Can you work these out from the model? Positions are in its coordinate system, mm. Face numbers are marked on the shaded views. A direction names the side the tool comes from. Round coordinates to 2 decimals unless told otherwise and drop trailing zeros. Order: outer loops, then holes, each group sorted by start corner. A loop starts at its lowest first (then second) coordinate and runs counter-clockwise, first axis right, second up. Notation, with made-up numbers: M 30,26.5 L 70,26.5 A18 cw 70,35.5 Z; hole C 30,11 d10. An arc over 180 degrees is marked long. Answer as a JSON object with one key per item and string values. Group by question number.
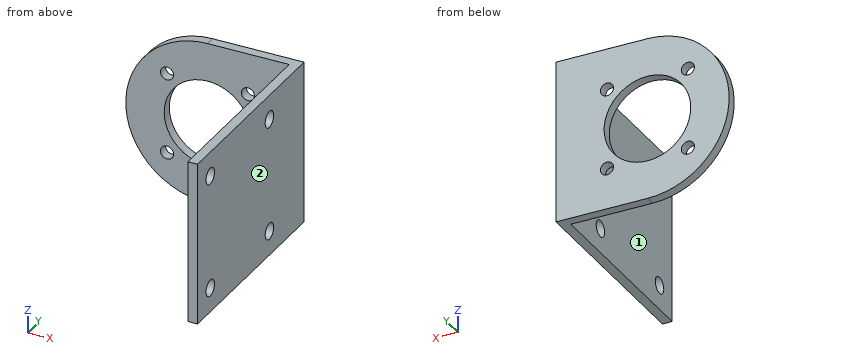
Autodesk Inventor part; units mm, degrees
ref_plane "YZ Plane" through (0, 0, 0) normal (1, 0, 0) x (0, 1, 0)
ref_plane "XZ Plane" through (0, 0, 0) normal (0, 1, 0) x (-1, 0, 0)
ref_plane "XY Plane" through (0, 0, 0) normal (0, 0, 1) x (1, 0, 0)
sketch "Sketch1" plane through (0, 0, 0) normal (0, 1, 0) x (-1, 0, 0)
  circle A0 centre (0, 0) radius 13.25
  line L0 (0, 0) -> (12.3744, 12.3744) construction
  line L1 (0, 0) -> (17.5, 0) construction
  line L2 (0, 0) -> (-12.3744, -12.3744) construction
  line L3 (0, 0) -> (17.5, 0) construction
  circle A1 centre (-12.3744, -12.3744) radius 2
  circle A2 centre (12.3744, 12.3744) radius 2
  circle A3 centre (12.3744, -12.3744) radius 2
  circle A4 centre (-12.3744, 12.3744) radius 2
  circle A5 centre (0, 0) radius 17.5 construction
  arc A6 (0, -25) -> (0, 25) centre (0, 0) ccw
  line L4 (0, 25) -> (-25, 25)
  line L5 (-25, 25) -> (-25, -25)
  line L6 (-25, -25) -> (0, -25)
  line L7 (-25, 25) -> (-28, 25)
  line L8 (-28, 25) -> (-28, -25)
  line L9 (-28, -25) -> (-25, -25)
  line L10 (-25, -25) -> (-25, 25)
  dimension "d0" = 26.5
  dimension "d1" = 17.5
  dimension "d2" = 45
  dimension "d3" = 17.5
  dimension "d4" = 135
  dimension "d5" = 4
  dimension "d6" = 4
  dimension "d7" = 50
  dimension "d10" = 3
extrude "Extrusion1" add sketch "Sketch1" along normal blind 3 contours L6 L5 L4 A6
extrude "Extrusion2" add sketch "Sketch1" along normal blind 3 and the other way blind 60 contours L9 L8 L7 L5
sketch "Sketch2" plane through (25, 0, -25) normal (-1, 0, 0) x (0, 0, 1)
  line L0 (50, -60) -> (50, 0) construction
  line L1 (0, -10) -> (50, -60) construction
  line L2 (7.5, -17.5) -> (42.5, -17.5) construction
  line L3 (42.5, -17.5) -> (42.5, -52.5) construction
  line L4 (42.5, -52.5) -> (7.5, -52.5) construction
  line L5 (7.5, -52.5) -> (7.5, -17.5) construction
  line L6 (7.5, -17.5) -> (42.5, -52.5) construction
  line L7 (42.5, -17.5) -> (7.5, -52.5) construction
  circle A0 centre (7.5, -17.5) radius 2.5
  circle A1 centre (42.5, -17.5) radius 2.5
  circle A2 centre (42.5, -52.5) radius 2.5
  circle A3 centre (7.5, -52.5) radius 2.5
  point P0 (25, 0)
  point P1 (25, -35)
  dimension "d15" = 35
  dimension "d16" = 35
  dimension "d17" = 5
extrude "Extrusion3" cut sketch "Sketch2" against normal blind 5
properties part number "Foundation-Motor-Mount" material "Steel, Mild"
1) If we section it at C-C on z = 17: Write out the boundary of the cut face in (x, y).
2) I need wall thicknesses on line 1 along Z through (x, y) = (0, 1); line 2 along Y through (x, z) = (17.5, 16); line 3 along X through (y, z) = (-13.5, 20). Which ranges of each line are inside material? Lowest first, please.
3) For pin 1 (6.5 mm diameter, centred on y = -17.5, z = -17.5, fed in from -X); pin 2 (3 mm diameter, centred on x = -12.37, z = -12.37, fed in from +Y); pin 3 (10 mm diameter, centred on x = 0.5, z = 16, fed in from -Y), each with a flat end and sliding along its axis, tell me the tip position at first contact or that it passes through.
4) If we section it at D-D on x = -4.5: Write out the boundary of the cut face in (y, z).
5) If we section it at A-A on z = -1: Write out the boundary of the cut face in (x, y), plus the area to 3 significant figures.
6) Which directions (+Z, -Z, +X, -X, +Y, -Y) give clear straight access to the entire face, cutting with the end or side of a thin tool? Please do the marked faces 1 and 2.
7) If we section it at B-B on y = -18.5: Write out the boundary of the cut face in (x, z).
Findings:
{
 "1": {"outline": "M -18.33,0 L 25,0 L 25,-15.05 L 28,-15.05 L 28,3 L -18.33,3 Z; M 25,-60 L 28,-60 L 28,-54.95 L 25,-54.95 Z; M 25,-50.05 L 28,-50.05 L 28,-19.95 L 25,-19.95 Z"},
 "2": {"line 1": "z = -25 to -13.25, 13.25 to 25", "line 2": "y = 0 to 3", "line 3": "x = 25 to 28"},
 "3": {"pin 1": "stops at x = 25", "pin 2": "passes through", "pin 3": "stops at y = 0"},
 "4": {"outline": "M 0,-24.59 L 3,-24.59 L 3,-12.46 L 0,-12.46 Z; M 0,12.46 L 3,12.46 L 3,24.59 L 0,24.59 Z"},
 "5": {"outline": "M -24.98,0 L -13.21,0 L -13.21,3 L -24.98,3 Z; M 13.21,0 L 25,0 L 25,-60 L 28,-60 L 28,3 L 13.21,3 Z", "area": "260 mm^2"},
 "6": {"face 1": "+Z, -Z, -X, -Y", "face 2": "+Z, -Z, +X, +Y, -Y"},
 "7": {"outline": "M 25,-25 L 28,-25 L 28,-19.79 L 25,-19.79 Z; M 25,-15.21 L 28,-15.21 L 28,15.21 L 25,15.21 Z; M 25,19.79 L 28,19.79 L 28,25 L 25,25 Z"}
}
